Check sheet for the modelled part. Datum: model origin and axes. Units: mm. Face numbers are marked on the shaded views. A direction names the side the tool comes from. Coordinates: 2 decimals unless noted, no trailing zeros. Loops run counter-clockwise (first coordinate to the right, second up) from the corner with the lowest first, then second, coordinate; pieces in that order, holes last.
```python
from build123d import *

# Parameters (mm, degrees)
BOSS_EXTRUDE1_DEPTH      = 60
BOSS_EXTRUDE1_DEPTH_BACK = 60
SKETCH2_W                = 30
SKETCH2_H                = 20
FILLET1_R                = 10


with BuildPart() as part:
    # Sketch1 → Revolve1 (revolve)
    with BuildSketch(Plane(origin=(0, 0, 0), x_dir=(0, 0, -1), z_dir=(1, 0, 0))):
        Polygon((0, 40.5), (0, 0), (11, 12), (11, 39.586753314), (10.816971936, 39.157197652), (10.816971936, 42.5), (0, 42.5), align=None)
    revolve(axis=Axis((0, 0, 0), (0, 1, 0)))


with BuildPart() as body_2:
    # Sketch1<3> → Revolve2 (revolve)
    with BuildSketch(Plane(origin=(0, 0, 0), x_dir=(0, 0, -1), z_dir=(1, 0, 0))):
        Polygon((24, 41.5), (24, 1), (35, 13), (35, 40.586753314), (35.621275123, 42.044847991), (35.621275123, 42.5), (24, 42.5), align=None)
    revolve(axis=Axis((0, 1, -24), (0, 1, 0)))


with BuildPart() as body_3:
    # Sketch1<4> → Revolve3 (revolve)
    with BuildSketch(Plane(origin=(0, 0, 0), x_dir=(0, 0, -1), z_dir=(1, 0, 0))):
        Polygon((48, 42.5), (48, 2), (59, 14), (59, 41.586753314), (59.389122501, 42.5), align=None)
    revolve(axis=Axis((0, 2, -48), (0, 1, 0)))


with BuildPart() as body_4:
    # Sketch1<5> → Revolve4 (revolve)
    with BuildSketch(Plane(origin=(0, 0, 0), x_dir=(0, 0, -1), z_dir=(1, 0, 0))):
        Polygon((-24, 39.501916964), (-24, -0.998083036), (-13, 11.001916964), (-13, 38.588670277), (-12.993341541, 38.604297273), (-12.993341541, 42.5), (-24, 42.5), align=None)
    revolve(axis=Axis((0, -0.998083036, 24), (0, 1, 0)))


with BuildPart() as body_5:
    # Sketch1<6> → Revolve5 (revolve)
    with BuildSketch(Plane(origin=(0, 0, 0), x_dir=(0, 0, -1), z_dir=(1, 0, 0))):
        Polygon((-48, 38.503833927), (-48, -1.996166073), (-37, 10.003833927), (-37, 37.590587241), (-36.686033209, 38.327448077), (-36.686033209, 42.5), (-48, 42.5), align=None)
    revolve(axis=Axis((0, -1.996166073, 48), (0, 1, 0)))


with BuildPart() as body_6:
    # Sketch2 → Boss-Extrude1 (new, two sides: drawn at the far end of the back side and taken through both)
    with BuildSketch(Plane.XY.offset(-BOSS_EXTRUDE1_DEPTH_BACK)):
        with Locations((0, 13)):
            Rectangle(SKETCH2_W, SKETCH2_H)
    extrude(amount=BOSS_EXTRUDE1_DEPTH + BOSS_EXTRUDE1_DEPTH_BACK)

    # Combine1: cut part, body 5, body 2, body 3, body 4
    add(part.part, mode=Mode.SUBTRACT)
    add(body_5.part, mode=Mode.SUBTRACT)
    add(body_2.part, mode=Mode.SUBTRACT)
    add(body_3.part, mode=Mode.SUBTRACT)
    add(body_4.part, mode=Mode.SUBTRACT)

    # Fillet1
    fillet1_edges = [body_6.edges().sort_by_distance(p)[0] for p in [
        (-15, 13, -60),
        (15, 13, -60),
        (15, 13, 60),
        (-15, 13, 60),
    ]]
    fillet(fillet1_edges, radius=FILLET1_R)


solid = body_6.part
```
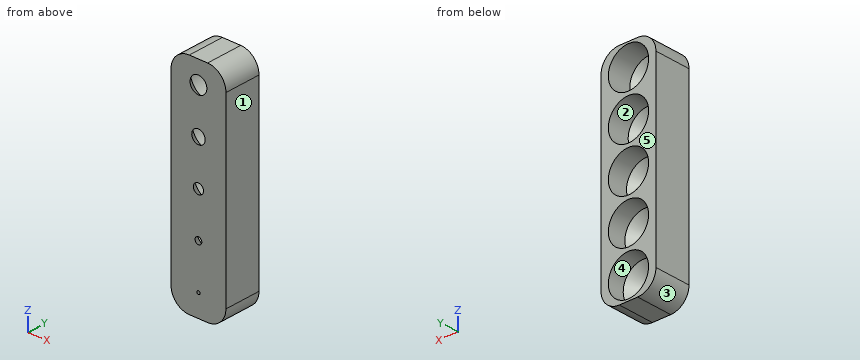
1) Section check D-D on z = 48. Enter the section's corners in (x, y).
Answer sheet:
outline: (-15, 3) - (-4.58, 3) - (-11, 10) - (-11, 23) - (-15, 23) - close; (4.58, 3) - (15, 3) - (15, 23) - (11, 23) - (11, 10) - close
2) Section check B-B on x = 0. Give the number of separate pieces and of enclosed holes in the cut face, plus the area to 3 significant figures.
Answer sheet:
separate pieces: 6
enclosed holes: 0
area: 580 mm2
3) Depth check by flat-ended pin: pin 1 (17.5 mm diameter, centred on x = 0, z = -24, fed in from +Y); pin 2 (3 mm diameter, centred on x = -3, z = -32.5, fed in from +Y). Enter the tip coordinate at first touch or a pass-through.
Answer sheet:
pin 1: stops at y = 10.55
pin 2: stops at y = 12.47
4) Mould release check, pull along Z, two halves, no side actions. Record for the marked faces 3, 4 and 5: +Z half, -Z half, draft (parallel to the pull), parting line (faces both ways), or undercut.
Answer sheet:
face 3: -Z half
face 4: undercut
face 5: draft
5) Set-up check for the marked faces 1 and 2: record each of +Z, -Z, +X, -X, +Y, -Y from which the full face is reachable in a straight line by a thin tool's end or side.
Answer sheet:
face 1: +Z, -Z, +X, +Y, -Y
face 2: +Y
6) Scan lines: line 1 (Z direction, x = 0, y = 18.75); line 2 (Z direction, x = -5, y = 7); line 3 (Z direction, x = 0, y = 5.75). Record each from-to range of solid material in increasing order.
Answer sheet:
line 1: z = -60 to -59, -37 to -35, -13 to -11, 11 to 13, 35 to 37, 59 to 60
line 2: z = -60 to -26.29, -21.71 to -4.02, 4.02 to 18.64, 29.36 to 41.44, 54.56 to 60
line 3: z = -60 to -51.44, -44.56 to -28.35, -19.65 to -5.27, 5.27 to 17.81, 30.19 to 40.9, 55.1 to 60
7) Section check C-C on y = 8.25. Enter the section's corners in (x, z) (1 decimal).
Answer sheet:
outline: (-15, -50) arc R10 ccw to (-5, -60) - (5, -60) arc R10 ccw to (15, -50) - (15, 50) arc R10 ccw to (5, 60) - (-5, 60) arc R10 ccw to (-15, 50) - close; hole circle Ø18.8 at (0, 48); hole circle Ø17 at (0, 24); hole circle Ø15.1 at (0, 0); hole circle Ø13.3 at (0, -24); hole circle Ø11.5 at (0, -48)
8) Section check A-A on z = 0. Enter the section's corners in (x, y), plus the area to 3 significant figures.
Answer sheet:
outline: (-15, 3) - (-2.75, 3) - (-11, 12) - (-11, 23) - (-15, 23) - close; (2.75, 3) - (15, 3) - (15, 23) - (11, 23) - (11, 12) - close
area: 234 mm2
